Verification items for the finished model (mm, model axes). A direction names the side the tool comes from. Round coordinates to 2 decimals unless told otherwise and drop trailing zeros. Write each loop counter-clockwise with the first axis right and the second up, starting at its lowest first coordinate (ties: lowest second). Pieces come first, ordered by that corner, then holes. Notation, with made-up numbers: M 63.5,89.5 L 78.5,89.5 A26 cw 78.5,126.5 Z; hole C -8,2.25 d10. An arc over 180 degrees is marked long. One line per question, with ' | ' between items.
from build123d import *

# Parameters (mm, degrees)
BOSS_EXTRUDE1_DEPTH = 285.75
CUT_EXTRUDE1_REACH  = 289.467
SKETCH2_R           = 2


with BuildPart() as part:
    # Sketch1 → Boss-Extrude1 (new body)
    with BuildSketch(Plane.XY):
        with BuildLine():
            Line((19.707457755, 0), (-10.292542245, 0))
            Line((-10.292542245, 0), (-10.292542245, 4))
            Line((-10.292542245, 4), (-1.292542245, 4))
            Line((-1.292542245, 4), (-1.292542245, 10.5))
            Line((-1.292542245, 10.5), (2.107457755, 17))
            ThreePointArc((2.107457755, 17), (4.707457755, 28.407402334), (7.307457755, 17))
            Line((7.307457755, 17), (10.707457755, 10.5))
            Line((10.707457755, 10.5), (10.707457755, 4))
            Line((10.707457755, 4), (19.707457755, 4))
            Line((19.707457755, 4), (19.707457755, 0))
        make_face()
    extrude(amount=BOSS_EXTRUDE1_DEPTH)

    # Sketch2 → Cut-Extrude1 (cut, up to next)
    with BuildSketch(Plane(origin=(0, 4, 0), x_dir=(1, 0, 0), z_dir=(0, 1, 0)), mode=Mode.PRIVATE) as cut_extrude1_sk1:
        with Locations(Location((-6.542542245, -50, 0), (0, 0, 270))):
            Circle(SKETCH2_R)
    cut_extrude1_tool1 = extrude(cut_extrude1_sk1.sketch, amount=-CUT_EXTRUDE1_REACH, mode=Mode.PRIVATE) & part.part
    # Sketch2 → Cut-Extrude1 (cut, up to next)
    with BuildSketch(Plane(origin=(0, 4, 0), x_dir=(1, 0, 0), z_dir=(0, 1, 0)), mode=Mode.PRIVATE) as cut_extrude1_sk2:
        with Locations(Location((15.957457755, -50, 0), (0, 0, 270))):
            Circle(SKETCH2_R)
    cut_extrude1_tool2 = extrude(cut_extrude1_sk2.sketch, amount=-CUT_EXTRUDE1_REACH, mode=Mode.PRIVATE) & part.part
    # Sketch2 → Cut-Extrude1 (cut, up to next)
    with BuildSketch(Plane(origin=(0, 4, 0), x_dir=(1, 0, 0), z_dir=(0, 1, 0)), mode=Mode.PRIVATE) as cut_extrude1_sk3:
        with Locations(Location((15.957457755, -150, 0), (0, 0, 270))):
            Circle(SKETCH2_R)
    cut_extrude1_tool3 = extrude(cut_extrude1_sk3.sketch, amount=-CUT_EXTRUDE1_REACH, mode=Mode.PRIVATE) & part.part
    # Sketch2 → Cut-Extrude1 (cut, up to next)
    with BuildSketch(Plane(origin=(0, 4, 0), x_dir=(1, 0, 0), z_dir=(0, 1, 0)), mode=Mode.PRIVATE) as cut_extrude1_sk4:
        with Locations(Location((-6.542542245, -150, 0), (0, 0, 270))):
            Circle(SKETCH2_R)
    cut_extrude1_tool4 = extrude(cut_extrude1_sk4.sketch, amount=-CUT_EXTRUDE1_REACH, mode=Mode.PRIVATE) & part.part
    # Sketch2 → Cut-Extrude1 (cut, up to next)
    with BuildSketch(Plane(origin=(0, 4, 0), x_dir=(1, 0, 0), z_dir=(0, 1, 0)), mode=Mode.PRIVATE) as cut_extrude1_sk5:
        with Locations(Location((15.957457755, -250, 0), (0, 0, 270))):
            Circle(SKETCH2_R)
    cut_extrude1_tool5 = extrude(cut_extrude1_sk5.sketch, amount=-CUT_EXTRUDE1_REACH, mode=Mode.PRIVATE) & part.part
    # Sketch2 → Cut-Extrude1 (cut, up to next)
    with BuildSketch(Plane(origin=(0, 4, 0), x_dir=(1, 0, 0), z_dir=(0, 1, 0)), mode=Mode.PRIVATE) as cut_extrude1_sk6:
        with Locations(Location((-6.542542245, -250, 0), (0, 0, 270))):
            Circle(SKETCH2_R)
    cut_extrude1_tool6 = extrude(cut_extrude1_sk6.sketch, amount=-CUT_EXTRUDE1_REACH, mode=Mode.PRIVATE) & part.part
    add(cut_extrude1_tool1.solids().sort_by_distance((-6.542542, 4, 50))[0], mode=Mode.SUBTRACT)
    add(cut_extrude1_tool2.solids().sort_by_distance((15.957458, 4, 50))[0], mode=Mode.SUBTRACT)
    add(cut_extrude1_tool3.solids().sort_by_distance((15.957458, 4, 150))[0], mode=Mode.SUBTRACT)
    add(cut_extrude1_tool4.solids().sort_by_distance((-6.542542, 4, 150))[0], mode=Mode.SUBTRACT)
    add(cut_extrude1_tool5.solids().sort_by_distance((15.957458, 4, 250))[0], mode=Mode.SUBTRACT)
    add(cut_extrude1_tool6.solids().sort_by_distance((-6.542542, 4, 250))[0], mode=Mode.SUBTRACT)


solid = part.part
1. Section check C-C, the plane y = 20.5. Record the cut outline in (x, z).
Results:
outline: M -0.98,0 L 10.4,0 L 10.4,285.75 L -0.98,285.75 Z
2. Thickness scan on line 1 (X direction, y = 1.75, z = 50); line 2 (Y direction, x = 16.25, z = 274); line 3 (Y direction, x = 5.5, z = 68.5). Record the ranges inside material, lowest first.
Results:
line 1: x = -10.29 to -8.54, -4.54 to 13.96, 17.96 to 19.71 | line 2: y = 0 to 4 | line 3: y = 0 to 28.35
3. Mould release check, pull along Y, two halves, no side actions. Record for faces 6 (the face through (-6, 4, 141)), 7 (the face through (8.98, 13.8, 140.87)), 8 (the face through (5, 0, 141)): pulls with the +Y half, pulls with the -Y half, needs draft (parallel to the pull), parting line crosses it, or undercut.
Results:
face 6: pulls with the +Y half | face 7: undercut | face 8: pulls with the -Y half
4. Section check B-B, the plane y = 8. Record the cut outline in (x, z), then the cut area to 3 significant figures.
Results:
outline: M -1.29,0 L 10.71,0 L 10.71,285.75 L -1.29,285.75 Z | area: 3,430 mm2
5. Go/stop test with flat-tipped pins: P1, Ø5, axis at y = 7, z = 96.5, coming from the +X side; P2, Ø7, axis at y = 8, z = 106.5, coming from the -X side; P3, Ø5, axis at x = -2.5, z = 224, coming from the +Y side. Record where each tip stops, or that it passes through.
Results:
P1: stops at x = 10.71 | P2: stops at x = -1.29 | P3: stops at y = 26.13
6. Tool access check on faces 1 (the face through (5, 11, 285.75)), 2 (the face through (5, 11, 0)), 3 (the face through (0.38, 13.7, 140.87)), 4 (the face through (-1.293, 7, 141)), 5 (the face through (15, 4, 141)). Record the directions out of +Z, -Z, +X, -X, +Y, -Y that give a thin tool (end or side, any length) a straight path to the whole face; none if there is none.
Results:
face 1: +Z, +X, -X, +Y, -Y | face 2: -Z, +X, -X, +Y, -Y | face 3: +Z, -Z, -X | face 4: +Z, -Z, -X, +Y | face 5: +Z, -Z, +X, +Y
7. Section check A-A, the plane z = 181. Record the cut outline in (x, y).
Results:
outline: M -10.29,0 L 19.71,0 L 19.71,4 L 10.71,4 L 10.71,10.5 L 7.31,17 A6 ccw long 2.11,17 L -1.29,10.5 L -1.29,4 L -10.29,4 Z
